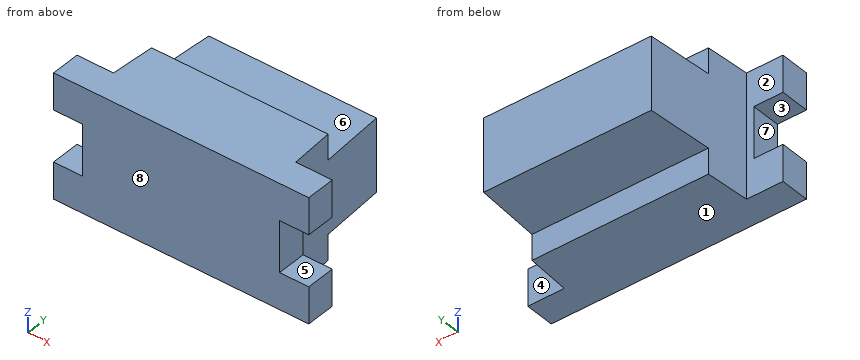
from build123d import *

# Parameters (mm, degrees)
BOSS_EXTRUDE1_DEPTH      = 17
BOSS_EXTRUDE1_DEPTH_BACK = 17
BOSS_EXTRUDE2_DEPTH      = 10
BOSS_EXTRUDE2_DEPTH_BACK = 10
SKETCH3_W                = 14
SKETCH3_H                = 8
CUT_EXTRUDE1_DEPTH       = 8
SKETCH4_W                = 14
SKETCH4_H                = 8
CUT_EXTRUDE2_DEPTH       = 8


with BuildPart() as part:
    # Sketch1 → Boss-Extrude1 (new, two sides: drawn at the far end of the back side and taken through both)
    with BuildSketch(Plane.XY.offset(-BOSS_EXTRUDE1_DEPTH_BACK)):
        Polygon((-37.863126543, -10.682367572), (-38.663126543, -22.682367572), (-48.663126543, -22.682367572), (-48.663126543, -30.682367572), (21.336873457, -30.682367572), (21.336873457, -22.682367572), (11.336873457, -22.682367572), (10.536873457, -10.682367572), align=None)
    extrude(amount=BOSS_EXTRUDE1_DEPTH + BOSS_EXTRUDE1_DEPTH_BACK)

    # Sketch1<3> → Boss-Extrude2 (add, two sides: drawn at the far end of the back side and taken through both)
    with BuildSketch(Plane.XY.offset(-BOSS_EXTRUDE2_DEPTH_BACK)):
        Polygon((-36.663126543, 7.317632428), (-37.863126543, -10.682367572), (10.536873457, -10.682367572), (9.336873457, 7.317632428), align=None)
    extrude(amount=BOSS_EXTRUDE2_DEPTH + BOSS_EXTRUDE2_DEPTH_BACK)

    # Sketch3 → Cut-Extrude1 (cut)
    with BuildSketch(Plane(origin=(21.336873457, 0, 0), x_dir=(0, 0, -1), z_dir=(1, 0, 0))):
        with Locations((0, -26.682367572)):
            Rectangle(SKETCH3_W, SKETCH3_H)
    extrude(amount=-CUT_EXTRUDE1_DEPTH, mode=Mode.SUBTRACT)

    # Sketch4 → Cut-Extrude2 (cut)
    with BuildSketch(Plane.ZY.offset(48.663126543)):
        with Locations((0, -26.682367572)):
            Rectangle(SKETCH4_W, SKETCH4_H)
    extrude(amount=-CUT_EXTRUDE2_DEPTH, mode=Mode.SUBTRACT)


solid = part.part
Can you work these out from the model? Positions are in its coordinate system, mm. Face numbers are marked on the shaded views. A direction names the side the tool comes from. Round coordinates to 2 decimals unless told otherwise and drop trailing zeros. Write each loop counter-clockwise with the first axis right and the second up, starting at its lowest first coordinate (ties: lowest second). Pieces come first, ordered by that corner, then holes. Notation, with made-up numbers: (67, 1) -> (99, 1) arc R31 cw to (99, 25) -> close; hole circle Ø9 at (-1.5, 70). An arc over 180 degrees is marked (long way). Use one line per item in the form item = value. Start each with the question number.
Q1. We'd pull the mould along Z, two halves only. Please class the marked faces 6, 7 and 8: +Z half, -Z half, draft (parallel to the pull), parting line (faces both ways), or undercut.
Q2. Imagine slicing it at A-A (z = 8.5). Please give me the cut outline in (x, y).
Q3. Imagine slicing it at B-B (x = 4). Please give me the cut outline in (y, z).
Q4. Imagine slicing it at D-D (y = 3). Please give me the cut outline in (x, z).
Q5. I'm going to push flat-ended pins straight in: P1, Ø14.5, axis at x = -6.5, y = -1, coming from the +Z side; P2, Ø10, axis at y = -7, z = -3.5, coming from the -X side; P3, Ø2, axis at x = -23, z = 13, coming from the +Y side; P4, Ø5, axis at x = 12.5, y = -22, coming from the +Z side. Where does each tip first touch, or does it pass through?
Q6. If I drill on probe 1 along Z at (x, y) = (18.5, -29); probe 2 along Z at (x, y) = (8.5, -6); probe 3 along Y at (x, z) = (-14.5, 13), over which ranges is the centre line in solid material (lowest first)? Write a range as [from, to].
Q7. Which directions (+Z, -Z, +X, -X, +Y, -Y) give clear straight access to the entire face, cutting with the end or side of a thin tool? Please do the marked faces 1, 2, 3, 4 and 5.
Q8. Imagine slicing it at C-C (y = -27). Please give me the cut outline in (x, z).
Worked out:
q1.face_6 = +Z half
q1.face_7 = undercut
q1.face_8 = draft
q2.outline = (-48.66, -30.68) -> (21.34, -30.68) -> (21.34, -22.68) -> (11.34, -22.68) -> (9.34, 7.32) -> (-36.66, 7.32) -> (-38.66, -22.68) -> (-48.66, -22.68) -> close
q3.outline = (-30.68, -17) -> (-10.68, -17) -> (-10.68, -10) -> (7.32, -10) -> (7.32, 10) -> (-10.68, 10) -> (-10.68, 17) -> (-30.68, 17) -> close
q4.outline = (-36.95, -10) -> (9.62, -10) -> (9.62, 10) -> (-36.95, 10) -> close
q5.P1 = 10
q5.P2 = -37.95
q5.P3 = -10.68
q5.P4 = 17
q6.probe_1 = [-17, -7], [7, 17]
q6.probe_2 = [-10, 10]
q6.probe_3 = [-30.68, -10.68]
q7.face_1 = -Z, +X, -X, +Y, -Y
q7.face_2 = +Z, -Z, -X, +Y
q7.face_3 = -X, +Y, -Y
q7.face_4 = +Z, -Z, +X, +Y
q7.face_5 = +X, +Y, -Y
q8.outline = (-48.66, -17) -> (21.34, -17) -> (21.34, -7) -> (13.34, -7) -> (13.34, 7) -> (21.34, 7) -> (21.34, 17) -> (-48.66, 17) -> (-48.66, 7) -> (-40.66, 7) -> (-40.66, -7) -> (-48.66, -7) -> close
